The figure shows three views and two pictorial views of one solid part (mm, origin at its lowest corner). Answer the questions. A direction names the side the tool comes from. Give positions to 0.01 mm unless a question says otherwise; leave off trailing zeros. Loops run counter-clockwise (first coordinate to the right, second up) from the corner with the lowest first, then second, coordinate; pieces in that order, holes last. Notation, with made-up numbers: (36, 45) - (83, 45) arc R9 cw to (83, 59) - close; hole circle Ø9 at (7, 49.25). An arc over 180 degrees is marked (long way). Write item = value, one per line.
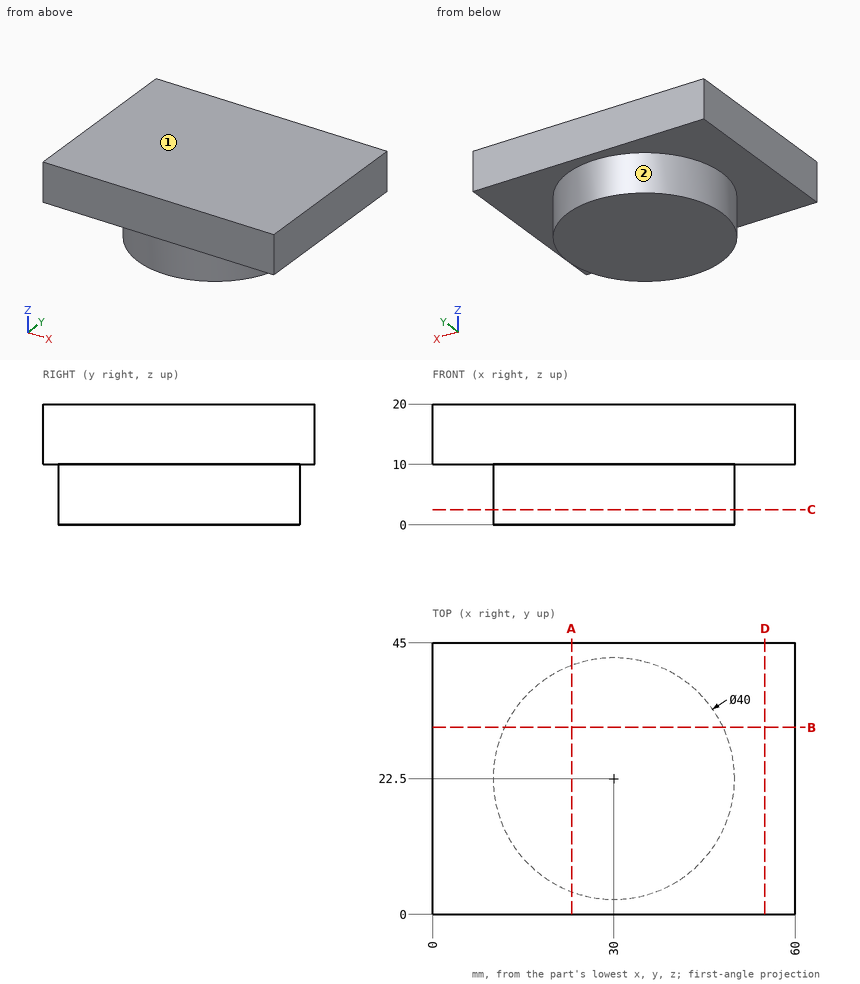
1) A cutting plane is placed at D-D on x = 55. Determine the outline of the cut face in (y, z), then the cut area to 3 significant figures.
Output:
outline = (0, 10) - (45, 10) - (45, 20) - (0, 20) - close
area = 450 mm²
2) A tool of negligible diameter and unlimited length cuts with its end or side. For the marked faces 1 and 2, from which of +Z, -Z, +X, -X, +Y, -Y can it reach the whole face along a straight path? Write none if from no direction.
Output:
face_1 = +Z, +X, -X, +Y, -Y
face_2 = -Z
3) A cutting plane is placed at B-B on y = 31. Determine the outline of the cut face in (x, z), then the cut area to 3 significant figures.
Output:
outline = (0, 10) - (11.9, 10) - (11.9, 0) - (48.1, 0) - (48.1, 10) - (60, 10) - (60, 20) - (0, 20) - close
area = 962 mm²
4) Each of these flat-tipped pins is pushed along its axis until it touches: P1, Ø2, axis at x = 44, z = 2, coming from the +Y side; P2, Ø6, axis at x = 43.5, z = 6.5, coming from the -Y side; P3, Ø4, axis at x = 42.5, z = 3.5, coming from the +Y side. Where does it stop, or does it pass through?
Output:
P1 = 37.7
P2 = 5.48
P3 = 39.52
5) Find the intervals of material crossed by probe 1 along Z at (x, y) = (38.5, 43.5); probe 2 along Y at (x, z) = (17, 4.5); probe 3 along X at (y, z) = (14, 5.5), in increasing order.
Output:
probe_1 = 10 to 20
probe_2 = 7.3 to 37.7
probe_3 = 11.9 to 48.1
6) A cutting plane is placed at A-A on x = 23. Determine the outline of the cut face in (y, z) (3 decimals).
Output:
outline = (0, 10) - (3.765, 10) - (3.765, 0) - (41.235, 0) - (41.235, 10) - (45, 10) - (45, 20) - (0, 20) - close
7) A cutting plane is placed at C-C on z = 2.5. Determine the outline of the cut face in (x, y), then the cut area to 3 significant figures.
Output:
outline = circle Ø40 at (30, 22.5)
area = 1,260 mm²
